Build history of the part. All positions in model axes, mm. Face numbers are marked on the shaded views. Coordinates: 2 decimals unless noted, no trailing zeros. Order: outer loops, then holes, each group sorted by start corner. A loop starts at its lowest first (then second) coordinate and runs counter-clockwise, first axis right, second up. Notation, with made-up numbers: (54, 71) - (72, 71) arc R23 cw to (72, 80) - close; hole circle Ø2 at (39, -28). An arc over 180 degrees is marked (long way). Write each question's results on one line, items separated by ' | '.
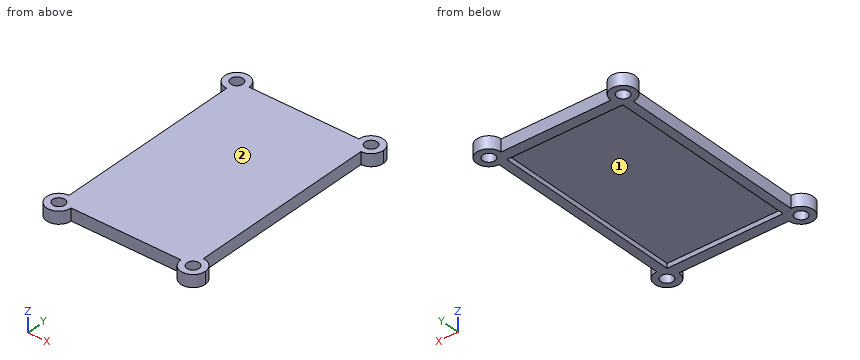
from build123d import *

# Parameters (mm, degrees)
F1_DEPTH = 4
F2_W     = 38
F2_H     = 63
F3_DEPTH = 1.5
F4_R     = 2
F5_DEPTH = 4


with BuildPart() as f1:
    # F0 (on Top) → F1 (new body)
    with BuildSketch(Plane.XY):
        with BuildLine():
            ThreePointArc((-22, 31), (-19.1715728753, 32.1715728753), (-18, 35))
            Line((-18, 35), (-22, 35))
            Line((-22, 35), (-22, 31))
        make_face()
        with BuildLine():
            Line((-22, 35), (-18, 35))
            ThreePointArc((-18, 35), (-24.8284271247, 37.8284271247), (-22, 31))
            Line((-22, 31), (-22, 35))
        make_face()
        with BuildLine():
            Line((18, 35), (-18, 35))
            ThreePointArc((-18, 35), (-19.1715728753, 32.1715728753), (-22, 31))
            Line((-22, 31), (-22, -31))
            ThreePointArc((-22, -31), (-19.1715728753, -32.1715728753), (-18, -35))
            Line((-18, -35), (18, -35))
            ThreePointArc((18, -35), (19.1715728753, -32.1715728753), (22, -31))
            Line((22, -31), (22, 31))
            ThreePointArc((22, 31), (19.1715728753, 32.1715728753), (18, 35))
        make_face()
        with BuildLine():
            ThreePointArc((26, 35), (22, 39), (18, 35))
            Line((18, 35), (22, 35))
            Line((22, 35), (22, 31))
            ThreePointArc((22, 31), (24.8284271247, 32.1715728753), (26, 35))
        make_face()
        with BuildLine():
            Line((22, 35), (18, 35))
            ThreePointArc((18, 35), (19.1715728753, 32.1715728753), (22, 31))
            Line((22, 31), (22, 35))
        make_face()
        with BuildLine():
            ThreePointArc((-18, -35), (-19.1715728753, -32.1715728753), (-22, -31))
            Line((-22, -31), (-22, -35))
            Line((-22, -35), (-18, -35))
        make_face()
        with BuildLine():
            Line((-22, -35), (-22, -31))
            ThreePointArc((-22, -31), (-24.8284271247, -37.8284271247), (-18, -35))
            Line((-18, -35), (-22, -35))
        make_face()
        with BuildLine():
            ThreePointArc((26, -35), (24.8284271247, -32.1715728753), (22, -31))
            Line((22, -31), (22, -35))
            Line((22, -35), (18, -35))
            ThreePointArc((18, -35), (22, -39), (26, -35))
        make_face()
        with BuildLine():
            Line((22, -35), (22, -31))
            ThreePointArc((22, -31), (19.1715728753, -32.1715728753), (18, -35))
            Line((18, -35), (22, -35))
        make_face()
    extrude(amount=F1_DEPTH)

    # F2 (on face) → F3 (cut)
    with BuildSketch(Plane(origin=(0, 0, 0), x_dir=(1, 0, 0), z_dir=(0, 0, -1))):
        Rectangle(F2_W, F2_H)
    extrude(amount=-F3_DEPTH, mode=Mode.SUBTRACT)

    # F4 (on face) → F5 (cut, through all)
    with BuildSketch(Plane(origin=(0, 0, 0), x_dir=(1, 0, 0), z_dir=(0, 0, -1))):
        with Locations((-22, 35)):
            Circle(F4_R)
        with Locations((22, 35)):
            Circle(F4_R)
        with Locations((-22, -35)):
            Circle(F4_R)
        with Locations((22, -35)):
            Circle(F4_R)
    extrude(amount=-F5_DEPTH, mode=Mode.SUBTRACT)


solid = f1.part
1. Band-saw the part on C-C on x = -14. Give the cut face in (y, z).
Solved:
outline: (-35, 0) - (-31.5, 0) - (-31.5, 1.5) - (31.5, 1.5) - (31.5, 0) - (35, 0) - (35, 4) - (-35, 4) - close
2. Probe line 1 (X direction, y = -20.5, z = 0.3); line 2 (Z direction, x = -15.5, y = -26.5); line 3 (Y direction, x = 4, z = 0.2). List the from-to ranges inside material, lowest first.
Solved:
line 1: x = -22 to -19, 19 to 22 | line 2: z = 1.5 to 4 | line 3: y = -35 to -31.5, 31.5 to 35
3. Band-saw the part on B-B on y = 19. Give the cut face in (x, z).
Solved:
outline: (-22, 0) - (-19, 0) - (-19, 1.5) - (19, 1.5) - (19, 0) - (22, 0) - (22, 4) - (-22, 4) - close
4. Drop flat-ended pins along their axis: pin 1 Ø1.5 at (x, y) = (-17.5, -20) entering from -Z; pin 2 Ø2 at (y, z) = (8, 2.5) entering from -X; pin 3 Ø1 at (x, z) = (-5, 2) entering from +Y. Give the stop position or say it passes through.
Solved:
pin 1: stops at z = 1.5 | pin 2: stops at x = -22 | pin 3: stops at y = 35
5. Two-plate mould, pull along X, no slides. Class the marked faces 1 and 2: +X half, -X half, draft (parallel to the pull), parting line (faces both ways), or undercut.
Solved:
face 1: undercut | face 2: draft
6. Band-saw the part on A-A on z = 2.85. Give the cut face in (x, y), then the cut area to 3 significant figures.
Solved:
outline: (-22, -31) arc R4 ccw (long way) to (-18, -35) - (18, -35) arc R4 ccw (long way) to (22, -31) - (22, 31) arc R4 ccw (long way) to (18, 35) - (-18, 35) arc R4 ccw (long way) to (-22, 31) - close; hole circle Ø4 at (-22, -35); hole circle Ø4 at (-22, 35); hole circle Ø4 at (22, -35); hole circle Ø4 at (22, 35) | area: 3,180 mm2
